Here's how the part is built. I have some questions about the finished solid (model axes, mm). A direction names the side the tool comes from. Round coordinates to 2 decimals unless told otherwise and drop trailing zeros. Loops run counter-clockwise (first coordinate to the right, second up) from the corner with the lowest first, then second, coordinate; pieces in that order, holes last. Notation, with made-up numbers: M 53,-18.5 L 105,-18.5 A29 ccw 105,9.5 Z; hole C 88.5,19 d8. An arc over 180 degrees is marked long. Answer as CSV lines item,"result".
```python
from build123d import *

# Parameters (mm, degrees)
REVOLVE1_ANGLE = 1


with BuildPart() as part:
    # Sketch4 → Revolve1 (revolve)
    with BuildSketch(Plane.XY):
        with BuildLine():
            Line((0, 0), (2.0574, 0))
            ThreePointArc((2.0574, 0), (3.673846102, 0.669553898), (4.3434, 2.286))
            Line((4.3434, 2.286), (4.3434, 3.2512))
            ThreePointArc((4.3434, 3.2512), (2.230011235, 5.623001416), (-0.368814742, 3.795993597))
            Line((-0.368814742, 3.795993597), (-1.27, 2.160242822))
            Line((-1.27, 2.160242822), (-1.27, 1.27))
            ThreePointArc((-1.27, 1.27), (-0.898025612, 0.371974388), (0, 0))
        make_face()
    revolve(axis=Axis((-132.03841004, 8.384500911, 0), (0, -1, 0)), revolution_arc=REVOLVE1_ANGLE)


solid = part.part
```
1. I want a section at B-B, the plane y = 1.7. Please give me the cut outline in (x, z).
Evaluation:
outline,"M -1.29,2.28 A130.77 cw -1.27,0 L 4.27,0 A136.31 ccw 4.25,2.38 Z"
2. I want a section at A-A, the plane y = 4.9. Please give me the cut outline in (x, z), and give its area (3 significant figures).
Evaluation:
outline,"M 0.21,2.31 A132.27 cw 0.23,0 L 3.68,0 A135.72 ccw 3.66,2.37 Z"
area,"8.08 mm²"
3. Which directions (+Z, -Z, +X, -X, +Y, -Y) give clear straight access to the entire face, cutting with the end or side of a thin tool? Please do faces 1 (the cylindrical face through (4.34, 2.78, 1.17)), 2 (the conical face through (-0.83, 2.97, 1.13)), 3 (the flat face through (1, 0, 1)), 4 (the cylindrical face through (-1.275, 1.709, 1.125)), 5 (the flat face through (1, 3, 0)).
Evaluation:
face 1,"+Z, +X, +Y, -Y"
face 2,"-Z, -X, +Y"
face 3,"+Z, -Z, +X, -X, -Y"
face 4,"-Z, -X, +Y, -Y"
face 5,"-Z, +X, -X, +Y, -Y"
4. For P1, Ø1, axis at y = 2, z = 1.5, coming from the +X side; P2, Ø1, axis at x = 3.5, y = 1, coming from the -Z side, each with a flat end and sliding along its axis, tell me the tip position at first contact or that it passes through.
Evaluation:
P1,"stops at x = 4.34"
P2,"stops at z = 0"
5. If I drill on line 1 (Z direction, x = -0.45, y = 1.4); line 2 (Y direction, x = 0, z = 0.5); line 3 (X direction, y = 2.15, z = 0.4), over which ranges is the centre line in solid material (lowest first)? Write a range as [from, to].
Evaluation:
line 1,"z = [0, 2.3]"
line 2,"y = [0, 4.62]"
line 3,"x = [-1.27, 4.34]"
